Could you check a few things on this model? Use its own coordinates, in mm. Give positions to 0.01 mm unless a question says otherwise; leave off trailing zeros. One line per item, written item: value.
```python
from build123d import *

# Parameters (mm, degrees)
SKETCH_1_R      = 3.4
EXTRUDE_1_DEPTH = 1000


with BuildPart() as part:
    # 草图1 → 凸台-拉伸1 (new body)
    with BuildSketch(Plane.XY):
        with BuildLine():
            Line((-11.148233949, 14.802957359), (-21.548233949, 14.802957359))
            ThreePointArc((-21.548233949, 14.802957359), (-24.730214465, 13.484937874), (-26.048233949, 10.302957359))
            Line((-26.048233949, 10.302957359), (-26.048233949, -0.097042641))
            Line((-26.048233949, -0.097042641), (-25.548233949, -0.097042641))
            ThreePointArc((-25.548233949, -0.097042641), (-25.194680559, -0.24348925), (-25.048233949, -0.597042641))
            Line((-25.048233949, -0.597042641), (-25.048233949, -1.097042641))
            Line((-25.048233949, -1.097042641), (-23.048233949, -1.097042641))
            Line((-23.048233949, -1.097042641), (-23.048233949, -0.097042641))
            Line((-23.048233949, -0.097042641), (-25.048233949, -0.097042641))
            Line((-25.048233949, -0.097042641), (-25.048233949, 5.202957359))
            Line((-25.048233949, 5.202957359), (-17.508894121, 5.202957359))
            Line((-17.508894121, 5.202957359), (-11.248233949, -1.057702813))
            Line((-11.248233949, -1.057702813), (-11.248233949, -9.336382469))
            Line((-11.248233949, -9.336382469), (-17.508894121, -15.597042641))
            Line((-17.508894121, -15.597042641), (-25.048233949, -15.597042641))
            Line((-25.048233949, -15.597042641), (-25.048233949, -10.797042641))
            ThreePointArc((-25.048233949, -10.797042641), (-24.90178734, -10.44348925), (-24.548233949, -10.297042641))
            Line((-24.548233949, -10.297042641), (-23.048233949, -10.297042641))
            Line((-23.048233949, -10.297042641), (-23.048233949, -9.297042641))
            Line((-23.048233949, -9.297042641), (-25.048233949, -9.297042641))
            Line((-25.048233949, -9.297042641), (-25.048233949, -9.797042641))
            ThreePointArc((-25.048233949, -9.797042641), (-25.194680559, -10.150596032), (-25.548233949, -10.297042641))
            Line((-25.548233949, -10.297042641), (-26.048233949, -10.297042641))
            Line((-26.048233949, -10.297042641), (-26.048233949, -20.697042641))
            ThreePointArc((-26.048233949, -20.697042641), (-24.730214465, -23.879023156), (-21.548233949, -25.197042641))
            Line((-21.548233949, -25.197042641), (-11.148233949, -25.197042641))
            Line((-11.148233949, -25.197042641), (-11.148233949, -24.697042641))
            ThreePointArc((-11.148233949, -24.697042641), (-11.00178734, -24.34348925), (-10.648233949, -24.197042641))
            Line((-10.648233949, -24.197042641), (-10.148233949, -24.197042641))
            Line((-10.148233949, -24.197042641), (-10.148233949, -22.197042641))
            Line((-10.148233949, -22.197042641), (-11.148233949, -22.197042641))
            Line((-11.148233949, -22.197042641), (-11.148233949, -23.697042641))
            ThreePointArc((-11.148233949, -23.697042641), (-11.294680559, -24.050596032), (-11.648233949, -24.197042641))
            Line((-11.648233949, -24.197042641), (-16.448233949, -24.197042641))
            Line((-16.448233949, -24.197042641), (-16.448233949, -16.657702813))
            Line((-16.448233949, -16.657702813), (-10.187573777, -10.397042641))
            Line((-10.187573777, -10.397042641), (-1.908894121, -10.397042641))
            Line((-1.908894121, -10.397042641), (4.351766051, -16.657702813))
            Line((4.351766051, -16.657702813), (4.351766051, -24.197042641))
            Line((4.351766051, -24.197042641), (-0.448233949, -24.197042641))
            ThreePointArc((-0.448233949, -24.197042641), (-0.80178734, -24.050596032), (-0.948233949, -23.697042641))
            Line((-0.948233949, -23.697042641), (-0.948233949, -22.197042641))
            Line((-0.948233949, -22.197042641), (-1.948233949, -22.197042641))
            Line((-1.948233949, -22.197042641), (-1.948233949, -24.197042641))
            Line((-1.948233949, -24.197042641), (-1.448233949, -24.197042641))
            ThreePointArc((-1.448233949, -24.197042641), (-1.094680559, -24.34348925), (-0.948233949, -24.697042641))
            Line((-0.948233949, -24.697042641), (-0.948233949, -25.197042641))
            Line((-0.948233949, -25.197042641), (9.451766051, -25.197042641))
            ThreePointArc((9.451766051, -25.197042641), (12.633746566, -23.879023156), (13.951766051, -20.697042641))
            Line((13.951766051, -20.697042641), (13.951766051, -10.297042641))
            Line((13.951766051, -10.297042641), (13.451766051, -10.297042641))
            ThreePointArc((13.451766051, -10.297042641), (13.09821266, -10.150596032), (12.951766051, -9.797042641))
            Line((12.951766051, -9.797042641), (12.951766051, -9.297042641))
            Line((12.951766051, -9.297042641), (10.951766051, -9.297042641))
            Line((10.951766051, -9.297042641), (10.951766051, -10.297042641))
            Line((10.951766051, -10.297042641), (12.451766051, -10.297042641))
            ThreePointArc((12.451766051, -10.297042641), (12.805319441, -10.44348925), (12.951766051, -10.797042641))
            Line((12.951766051, -10.797042641), (12.951766051, -15.597042641))
            Line((12.951766051, -15.597042641), (5.412426223, -15.597042641))
            Line((5.412426223, -15.597042641), (-0.848233949, -9.336382469))
            Line((-0.848233949, -9.336382469), (-0.848233949, -1.057702813))
            Line((-0.848233949, -1.057702813), (5.412426223, 5.202957359))
            Line((5.412426223, 5.202957359), (12.951766051, 5.202957359))
            Line((12.951766051, 5.202957359), (12.951766051, 0.402957359))
            ThreePointArc((12.951766051, 0.402957359), (12.805319441, 0.049403968), (12.451766051, -0.097042641))
            Line((12.451766051, -0.097042641), (10.951766051, -0.097042641))
            Line((10.951766051, -0.097042641), (10.951766051, -1.097042641))
            Line((10.951766051, -1.097042641), (12.951766051, -1.097042641))
            Line((12.951766051, -1.097042641), (12.951766051, -0.597042641))
            ThreePointArc((12.951766051, -0.597042641), (13.09821266, -0.24348925), (13.451766051, -0.097042641))
            Line((13.451766051, -0.097042641), (13.951766051, -0.097042641))
            Line((13.951766051, -0.097042641), (13.951766051, 10.302957359))
            ThreePointArc((13.951766051, 10.302957359), (12.633746566, 13.484937874), (9.451766051, 14.802957359))
            Line((9.451766051, 14.802957359), (-0.948233949, 14.802957359))
            Line((-0.948233949, 14.802957359), (-0.948233949, 14.302957359))
            ThreePointArc((-0.948233949, 14.302957359), (-1.094680559, 13.949403968), (-1.448233949, 13.802957359))
            Line((-1.448233949, 13.802957359), (-1.948233949, 13.802957359))
            Line((-1.948233949, 13.802957359), (-1.948233949, 11.802957359))
            Line((-1.948233949, 11.802957359), (-0.948233949, 11.802957359))
            Line((-0.948233949, 11.802957359), (-0.948233949, 13.302957359))
            ThreePointArc((-0.948233949, 13.302957359), (-0.80178734, 13.65651075), (-0.448233949, 13.802957359))
            Line((-0.448233949, 13.802957359), (4.351766051, 13.802957359))
            Line((4.351766051, 13.802957359), (4.351766051, 6.263617531))
            Line((4.351766051, 6.263617531), (-1.908894121, 0.002957359))
            Line((-1.908894121, 0.002957359), (-10.187573777, 0.002957359))
            Line((-10.187573777, 0.002957359), (-16.448233949, 6.263617531))
            Line((-16.448233949, 6.263617531), (-16.448233949, 13.802957359))
            Line((-16.448233949, 13.802957359), (-11.648233949, 13.802957359))
            ThreePointArc((-11.648233949, 13.802957359), (-11.294680559, 13.65651075), (-11.148233949, 13.302957359))
            Line((-11.148233949, 13.302957359), (-11.148233949, 11.802957359))
            Line((-11.148233949, 11.802957359), (-10.148233949, 11.802957359))
            Line((-10.148233949, 11.802957359), (-10.148233949, 13.802957359))
            Line((-10.148233949, 13.802957359), (-10.648233949, 13.802957359))
            ThreePointArc((-10.648233949, 13.802957359), (-11.00178734, 13.949403968), (-11.148233949, 14.302957359))
            Line((-11.148233949, 14.302957359), (-11.148233949, 14.802957359))
        make_face()
        with Locations((-6.048233949, -5.197042641)):
            Circle(SKETCH_1_R, mode=Mode.SUBTRACT)
        with BuildLine():
            Line((-17.448233949, 13.802957359), (-21.548233949, 13.802957359))
            ThreePointArc((-21.548233949, 13.802957359), (-24.023107683, 12.777831093), (-25.048233949, 10.302957359))
            Line((-25.048233949, 10.302957359), (-25.048233949, 6.202957359))
            Line((-25.048233949, 6.202957359), (-17.448233949, 6.202957359))
            Line((-17.448233949, 6.202957359), (-17.448233949, 13.802957359))
        make_face(mode=Mode.SUBTRACT)
        with BuildLine():
            Line((5.351766051, 13.802957359), (9.451766051, 13.802957359))
            ThreePointArc((9.451766051, 13.802957359), (11.926639785, 12.777831093), (12.951766051, 10.302957359))
            Line((12.951766051, 10.302957359), (12.951766051, 6.202957359))
            Line((12.951766051, 6.202957359), (5.351766051, 6.202957359))
            Line((5.351766051, 6.202957359), (5.351766051, 13.802957359))
        make_face(mode=Mode.SUBTRACT)
        with BuildLine():
            Line((-17.448233949, -24.197042641), (-21.548233949, -24.197042641))
            ThreePointArc((-21.548233949, -24.197042641), (-24.023107683, -23.171916375), (-25.048233949, -20.697042641))
            Line((-25.048233949, -20.697042641), (-25.048233949, -16.597042641))
            Line((-25.048233949, -16.597042641), (-17.448233949, -16.597042641))
            Line((-17.448233949, -16.597042641), (-17.448233949, -24.197042641))
        make_face(mode=Mode.SUBTRACT)
        with BuildLine():
            Line((5.351766051, -24.197042641), (9.451766051, -24.197042641))
            ThreePointArc((9.451766051, -24.197042641), (11.926639785, -23.171916375), (12.951766051, -20.697042641))
            Line((12.951766051, -20.697042641), (12.951766051, -16.597042641))
            Line((12.951766051, -16.597042641), (5.351766051, -16.597042641))
            Line((5.351766051, -16.597042641), (5.351766051, -24.197042641))
        make_face(mode=Mode.SUBTRACT)
    extrude(amount=EXTRUDE_1_DEPTH)


solid = part.part
```
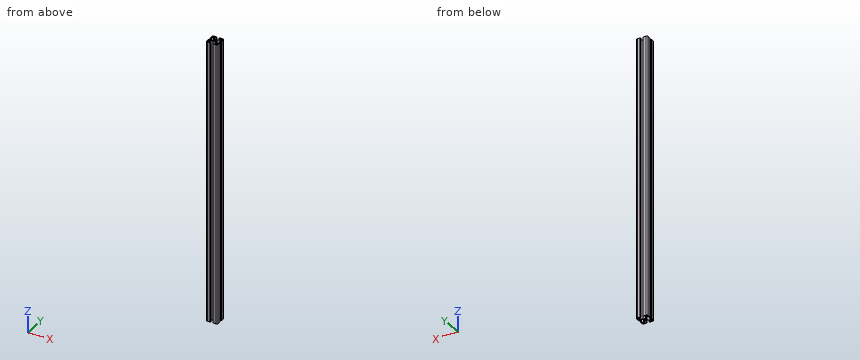
1) If we section it at A-A, the plane z = 356.5: Give the number of separate pieces and of enclosed holes in the cut face, then the cut area to 3 significant figures.
Outcome:
separate pieces: 1
enclosed holes: 5
area: 310 mm^2
2) Please list where these lines run through material, in increasing order: L1, parallel to Y at x = 11.5, z = 929.5; L2, parallel to X at y = -9.5, z = 548.5; L3, parallel to X at y = 8.5, z = 736. Write a range as from..to.
Outcome:
L1: y = -24.7..-23.54, -16.6..-15.6, -10.3..-9.3, -1.1..-0.1, 5.2..6.2, 13.14..14.31
L2: x = -25.05..-23.05, -11.41..-0.68, 10.95..12.95
L3: x = -26.05..-25.05, -17.45..-16.45, 4.35..5.35, 12.95..13.95
3) I'm going to push flat-ended pins straight in: pin 1 (4 mm diameter, centred on x = -6.5, z = 517.5, fed in from -Y); pin 2 (2 mm diameter, centred on x = -2, y = -20.5, fed in from -Z); pin 3 (4 mm diameter, centred on y = -4.5, z = 339, fed in from +X); pin 4 (1.6 mm diameter, centred on y = -23, z = 489.5, fed in from -X). Where does each tip first touch, or does it pass through?
Outcome:
pin 1: stops at y = -10.4
pin 2: passes through
pin 3: stops at x = -0.85
pin 4: stops at x = -25.79
